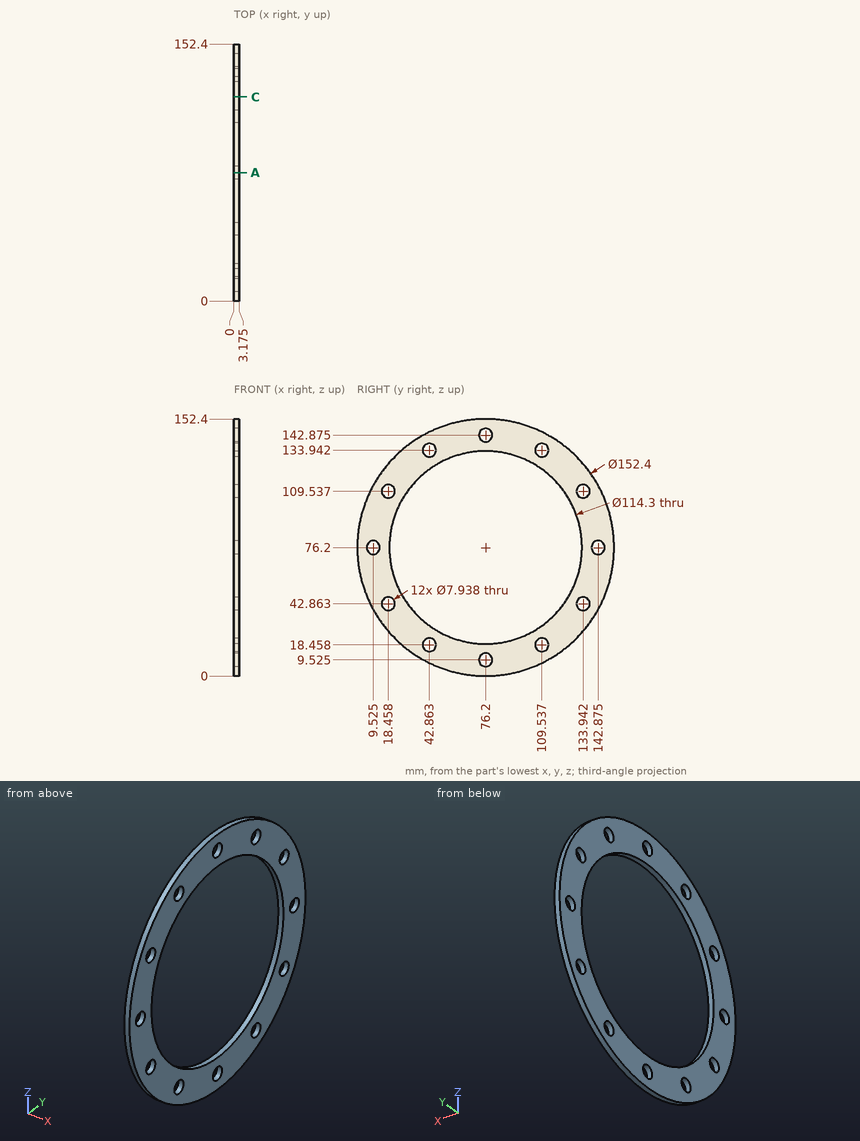
Part print with two shaded views. Sizes in mm from the minimum x, y, z corner. Coordinates: 2 decimals unless noted, no trailing zeros. Write each loop counter-clockwise with the first axis right and the second up, starting at its lowest first coordinate (ties: lowest second). Pieces come first, ordered by that corner, then holes. Notation, with made-up numbers: (-24.5, 53) - (31.5, 53) arc R29 ccw to (31.5, 87) - close; hole circle Ø7 at (-35.5, 30.25). An arc over 180 degrees is marked (long way). Put each result on its own line as item: value.
1. Band-saw the part on C-C (y = 121). Write the cut outline in (x, z) (1 decimal).
Final values:
outline: (0, 14.6) - (3.2, 14.6) - (3.2, 40.7) - (0, 40.7) - close; (0, 111.7) - (3.2, 111.7) - (3.2, 137.8) - (0, 137.8) - close
2. Probe line 1 along Z through (x, y) = (1.95, 76.2); line 2 along Y through (x, z) = (0.6, 17) (1 decimal); line 3 along Y through (x, z) = (0.6, 46) (1 decimal). List the from-to ranges inside material, lowest first. Write a range as [from, to].
Final values:
line 1: z = [0, 5.56], [13.49, 19.05], [133.35, 138.91], [146.84, 152.4]
line 2: y = [28.2, 39.2], [46.6, 105.8], [113.2, 124.2]
line 3: y = [6.2, 16], [20.9, 27.7], [124.7, 131.5], [136.4, 146.2]
3. Flat gauge pins, fed straight in: pin 1 Ø1.5 at (x, z) = (1.5, 115.5) entering from -Y; pin 2 Ø10.5 at (y, z) = (109.54, 18.46) entering from -X; pin 3 Ø6.5 at (y, z) = (42.86, 18.46) entering from -X; pin 4 Ø1 at (x, y) = (0.5, 90) entering from -Z. Where does each tip first touch, or does it go through?
Final values:
pin 1: stops at y = 10.47
pin 2: stops at x = 0
pin 3: passes through
pin 4: stops at z = 1.17
4. Band-saw the part on A-A (y = 76.2). Give the number of separate pieces and of enclosed holes in the cut face.
Final values:
separate pieces: 4
enclosed holes: 0
